Autodesk Fusion 360 part; units mm, degrees
sketch "Sketch1" plane through (0, 0, 0) normal (0, 0, 1) x (1, 0, 0)
  line L0 (16.12, 50) -> (16.12, -69.76)
  line L1 (16.12, -69.76) -> (80, -69.76)
  line L2 (80, -69.76) -> (80, 50)
  line L3 (80, 50) -> (75, 50)
  line L4 (75, 50) -> (75, -64.76)
  line L5 (75, -64.76) -> (21.12, -64.76)
  line L6 (21.12, -64.76) -> (21.12, 50)
  line L7 (21.12, 50) -> (16.12, 50)
  circle A0 centre (18.62, 47.5) radius 1.25
  circle A1 centre (77.5, 47.5) radius 1.25
  circle A2 centre (18.62, -67.26) radius 1.25
  circle A3 centre (77.5, -67.26) radius 1.25
  dimension "d9" = 5
  dimension "d10" = 5
  dimension "d11" = 5
  dimension "d12" = 119.76
  dimension "d13" = 63.88
  dimension "d16" = 2.5
  dimension "d17" = 2.5
  dimension "d18" = 2.5
  dimension "d19" = 2.5
  dimension "d20" = 2.5
  dimension "d21" = 2.5
  dimension "d22" = 2.5
  dimension "d23" = 2.5
  dimension "d24" = 2.5
  dimension "d25" = 2.5
  dimension "d26" = 2.5
  dimension "d27" = 2.5
  dimension "d39" = 114.76
extrude "Extrude2" add sketch "Sketch1" along normal blind 18
sketch "Sketch3" plane through (0, 50, 0) normal (0, 1, 0) x (-1, 0, 0)
  line L0 (-80, 0) -> (-75, 0)
  line L1 (-75, 0) -> (-75, 18)
  line L2 (-75, 18) -> (-80, 18)
  line L3 (-80, 18) -> (-80, 0)
  line L4 (-75, 10) -> (-76, 10)
  line L5 (-76, 10) -> (-76, 13)
  line L6 (-76, 13) -> (-75, 13)
  line L7 (-75, 13) -> (-75, 10)
  dimension "d34" = 3
  dimension "d35" = 1
  dimension "d36" = 5
extrude "Extrude3" cut sketch "Sketch3" against normal blind 115.76 contours L1 L4 L5 L6 L7
sketch "Sketch4" plane through (0, -64.76, 0) normal (0, 1, 0) x (-1, 0, 0)
  line L0 (-75, 0) -> (-21.12, 0)
  line L1 (-21.12, 0) -> (-21.12, 18)
  line L2 (-21.12, 18) -> (-75, 18)
  line L3 (-75, 18) -> (-75, 13)
  line L4 (-75, 13) -> (-75, 10)
  line L5 (-75, 10) -> (-75, 0)
  line L6 (-75, 13) -> (-21.12, 13)
  line L7 (-21.12, 13) -> (-21.12, 9)
  line L8 (-21.12, 9) -> (-75, 9)
  line L9 (-75, 9) -> (-75, 13)
extrude "Extrude4" cut sketch "Sketch4" against normal blind 1 contours L1 L4 L5 L6 L7 L8 L9
sketch "Sketch5" plane through (0, 50, 0) normal (0, 1, 0) x (-1, 0, 0)
  line L0 (-21.12, 0) -> (-16.12, 0)
  line L1 (-16.12, 0) -> (-16.12, 18)
  line L2 (-16.12, 18) -> (-21.12, 18)
  line L3 (-21.12, 18) -> (-21.12, 0)
  line L4 (-21.12, 13) -> (-20.12, 13)
  line L5 (-20.12, 13) -> (-20.12, 10)
  line L6 (-20.12, 10) -> (-21.12, 10)
  line L7 (-21.12, 10) -> (-21.12, 13)
  dimension "d42" = 3
  dimension "d43" = 5
  dimension "d44" = 1
extrude "Extrude5" cut sketch "Sketch5" against normal blind 115.76 contours L3 L4 L5 L6 L7
sketch "Sketch6" plane through (0, 0, 10) normal (0, 0, 1) x (-1, 0, 0)
  line L0 (-21.12, 65.76) -> (-21.12, -50)
  line L1 (-21.12, -50) -> (-20.12, -50)
  line L2 (-20.12, -50) -> (-20.12, 65.76)
  line L3 (-20.12, 65.76) -> (-21.12, 65.76)
  line L4 (-20.12, -50) -> (-21.12, -50)
  line L5 (-21.12, -50) -> (-21.12, -46)
  line L6 (-21.12, -46) -> (-20.12, -46)
  line L7 (-20.12, -46) -> (-20.12, -50)
  dimension "d47" = 4
extrude "Extrude6" add sketch "Sketch6" along normal blind 2 contours L0 L1 L2 L4 L5 L6 L7
sketch "Sketch7" plane through (0, 0, 10) normal (0, 0, 1) x (-1, 0, 0)
  line L0 (-20.12, 65.76) -> (-21.12, 65.76)
  line L1 (-75, -50) -> (-76, -50)
  line L2 (-76, -50) -> (-76, -46)
  line L3 (-76, -46) -> (-75, -46)
  line L4 (-75, -46) -> (-75, -50)
  line L5 (-21.12, -46) -> (-20.12, -46)
  line L6 (-20.12, -46) -> (-20.12, 65.76)
  line L7 (-21.12, 65.76) -> (-21.12, -46)
extrude "Extrude9" add 1 faces at (39.08, -65.0933, 9) along direction (0, 0, 1) blind 1
extrude "Extrude10" add 1 faces at (20.7867, 47.3333, 12) along direction (0, 0, 1) blind 1
extrude "Extrude11" add sketch "Sketch7" along normal blind 3 contours L1 L2 L3 L4
extrude "Extrude12" cut 1 faces at (20.4533, 46, 12) along direction (0, 1, 0) blind 1
extrude "Extrude13" cut 1 faces at (75.6667, 46, 11) along direction (0, 1, 0) blind 1
extrude "Extrude14" cut 1 faces at (77.057, -28.1733, 0) along direction (0, 0, 1) blind 5
extrude "Extrude7" [suppressed]
extrude "Extrude8" [suppressed]
Build history of the part. All positions in model axes, mm. A direction names the side the tool comes from. Round coordinates to 2 decimals unless told otherwise and drop trailing zeros. Write each loop counter-clockwise with the first axis right and the second up, starting at its lowest first coordinate (ties: lowest second). Pieces come first, ordered by that corner, then holes.
1) 3-axis set-ups, long thin cutter, end or side, ignore diameter. For faces 1 (the flat face through (20.12, -9, 12)), 2 (the flat face through (20, -23, 5)), 3 (the flat face through (48, -64.76, 15)): which of +Z, -Z, +X, -X, +Y, -Y reach the whole face in a straight line?
2) Pin check, flat tips, straight feed: pin 1 (4 mm diameter, centred on x = 50, z = 8.5, fed in from +Y); pin 2 (1.5 mm diameter, centred on x = 77.5, y = -67.26, fed in from +Z) (3 decimals). Stop position of each tip, or through.
3) Mould opens along X. For faces 4 (the flat face through (20, -23, 18)), 5 (the flat face through (48, -64.76, 7)), 6 (the flat face through (80, -11, 11)) say: +X half, -X half, draft (parallel to the pull), parting line (faces both ways), or undercut.
4) Drill centre lines: probe 1 along X at (y, z) = (-67.26, 15.5); probe 2 along Y at (x, z) = (18.62, 9.25); probe 3 along X at (y, z) = (-50.5, 8.75). Where is each one in solid material? Low to high.
5) Band-saw the part on C-C, the plane y = -67.26. List the corners of the cut face in (x, z).
6) Band-saw the part on B-B, the plane x = 77.5. List the corners of the cut face in (y, z).
7) Band-saw the part on A-A, the plane y = -16. List the corners of the cut face in (x, z).
8) Band-saw the part on D-D, the plane z = 15.25. List the corners of the cut face in (x, y).
Ans:
1. face 1: none
1. face 2: -Z, +X, -X, +Y, -Y
1. face 3: +Z, -Z, +Y
2. pin 1: stops at y = -64.76
2. pin 2: passes through
3. face 4: draft
3. face 5: undercut
3. face 6: +X half
4. probe 1: x = 16.12 to 17.37, 19.87 to 76.25, 78.75 to 80
4. probe 2: y = -69.76 to -68.51, -66.01 to 46.25, 48.75 to 50
4. probe 3: x = 16.12 to 21.12, 75 to 80
5. outline: (16.12, 5) - (17.37, 5) - (17.37, 18) - (16.12, 18) - close; (19.87, 5) - (76.25, 5) - (76.25, 18) - (19.87, 18) - close; (78.75, 5) - (80, 5) - (80, 18) - (78.75, 18) - close
6. outline: (-69.76, 5) - (-68.51, 5) - (-68.51, 18) - (-69.76, 18) - close; (-66.01, 5) - (46.25, 5) - (46.25, 18) - (-66.01, 18) - close; (48.75, 5) - (50, 5) - (50, 18) - (48.75, 18) - close
7. outline: (16.12, 5) - (21.12, 5) - (21.12, 10) - (20.12, 10) - (20.12, 13) - (21.12, 13) - (21.12, 18) - (16.12, 18) - close; (75, 5) - (80, 5) - (80, 18) - (75, 18) - (75, 13) - (76, 13) - (76, 10) - (75, 10) - close
8. outline: (16.12, -69.76) - (80, -69.76) - (80, 50) - (75, 50) - (75, -64.76) - (21.12, -64.76) - (21.12, 50) - (16.12, 50) - close; hole circle Ø2.5 at (18.62, -67.26); hole circle Ø2.5 at (18.62, 47.5); hole circle Ø2.5 at (77.5, -67.26); hole circle Ø2.5 at (77.5, 47.5)
